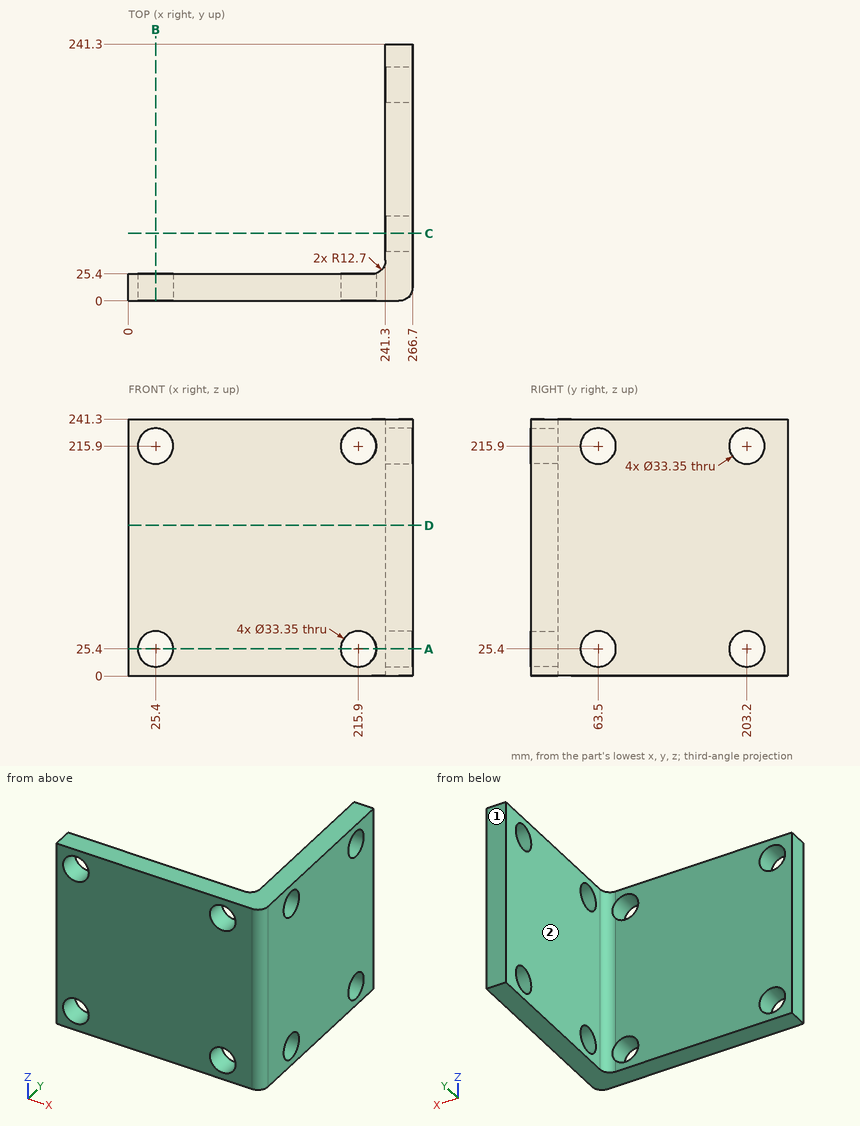
Answer from the drawing. Dimensions are ordinates in mm from the lowest x, y and z of the part. A direction names the side the tool comes from. Coordinates: 2 decimals unless noted, no trailing zeros. Write each loop counter-clockwise with the first axis right and the second up, starting at its lowest first coordinate (ties: lowest second). Pieces come first, ordered by that corner, then holes. Notation, with made-up numbers: (60, -26) - (118, -26) arc R19 cw to (118, -17) - close; hole circle Ø2 at (76.25, 46.25). An arc over 180 degrees is marked (long way). Return JSON: item names as keys, results as strings. Group by question number.
Q1. Find the intervals of material crossed by line 1 along Y through (x, z) = (254, 215); line 2 along Z through (x, y) = (215, 8); line 3 along Z through (x, y) = (215.9, 9.5) (1 decimal), in increasing order. Write a range as [from, to].
Q2. The part is cut by section C-C on y = 63.5. Write down the section's boundary in (x, z) (1 decimal), and give its area (4 significant figures).
Q3. The part is cut by section B-B on x = 25.4. Write down the section's boundary in (y, z) (1 decimal).
Q4. The part is cut by section A-A on z = 25.4. Write down the section's boundary in (x, y) (1 decimal), and give its area (3 significant figures).
Q5. Which of the six approach directions +Z, -Z, +X, -X, +Y, -Y give full straight-line access (tool end or side, diameter ignored) to the marked faces 1 and 2?
Q6. A flat-ended cylindrical pin translates along its axis: pin 1 Ø3 at (y, z) = (177, 180.5) entering from -X. Find the tip coordinate at first contact, or state that the pin passes through.
Q7. The part is cut by section D-D on z = 141.5. Write down the section's boundary in (x, y), and give its area (3 significant figures).
Evaluation:
{
 "1": {"line 1": "y = [0, 46.85], [80.15, 186.55], [219.85, 241.3]", "line 2": "z = [0, 8.75], [42.05, 199.25], [232.55, 241.3]", "line 3": "z = [0, 8.7], [42.1, 199.2], [232.6, 241.3]"},
 "2": {"outline": "(241.3, 0) - (266.7, 0) - (266.7, 8.7) - (241.3, 8.7) - close; (241.3, 42.1) - (266.7, 42.1) - (266.7, 199.2) - (241.3, 199.2) - close; (241.3, 232.6) - (266.7, 232.6) - (266.7, 241.3) - (241.3, 241.3) - close", "area": "4,435 mm2"},
 "3": {"outline": "(0, 0) - (25.4, 0) - (25.4, 8.7) - (0, 8.7) - close; (0, 42.1) - (25.4, 42.1) - (25.4, 199.2) - (0, 199.2) - close; (0, 232.6) - (25.4, 232.6) - (25.4, 241.3) - (0, 241.3) - close"},
 "4": {"outline": "(0, 0) - (8.7, 0) - (8.7, 25.4) - (0, 25.4) - close; (42.1, 0) - (199.2, 0) - (199.2, 25.4) - (42.1, 25.4) - close; (232.6, 0) - (254, 0) arc R12.7 ccw to (266.7, 12.7) - (266.7, 46.8) - (241.3, 46.8) - (241.3, 38.1) arc R12.7 cw to (232.6, 26) - close; (241.3, 80.2) - (266.7, 80.2) - (266.7, 186.5) - (241.3, 186.5) - close; (241.3, 219.9) - (266.7, 219.9) - (266.7, 241.3) - (241.3, 241.3) - close", "area": "8,870 mm2"},
 "5": {"face 1": "+Z, -Z, +X, -X, +Y", "face 2": "+Z, -Z, -X, +Y"},
 "6": {"pin 1": "stops at x = 241.3"},
 "7": {"outline": "(0, 0) - (254, 0) arc R12.7 ccw to (266.7, 12.7) - (266.7, 241.3) - (241.3, 241.3) - (241.3, 38.1) arc R12.7 cw to (228.6, 25.4) - (0, 25.4) - close", "area": "12,300 mm2"}
}
